Input: part model. Units: mm. Frame: model coordinates. Face numbers are marked on the shaded views. A direction names the side the tool comes from. Round coordinates to 2 decimals unless told otherwise and drop trailing zeros. Order: outer loops, then holes, each group sorted by start corner. A loop starts at its lowest first (then second) coordinate and runs counter-clockwise, first axis right, second up. Notation, with made-up numbers: M 74,-37.75 L 97,-37.75 A26 cw 97,-17.75 Z; hole C 57,60.25 d10. An arc over 180 degrees is marked long. One line per question, with ' | ' between items.
```python
from build123d import *

# Parameters (mm, degrees)
SKETCH_1_W         = 110
SKETCH_1_H         = 74
EXTRUDE_10_DEPTH   = 70
EXTRUDE_10_2_DEPTH = 70
EXTRUDE_10_3_DEPTH = 70
EXTRUDE_11_DEPTH   = 65
SKETCH_1_12_W      = 110
SKETCH_1_12_H      = 74
SKETCH_1_12_R      = 2
EXTRUDE_12_DEPTH   = 6


with BuildPart() as part:
    # Sketch 1 → Extrude 10 (new body)
    with BuildSketch(Plane.XY):
        Polygon((60.422680412, 44.278350515), (-55.577319588, 44.278350515), (-55.577319588, 38.278350515), (-55.577319588, -35.721649485), (-55.577319588, -41.721649485), (60.422680412, -41.721649485), (60.422680412, -35.721649485), (60.422680412, 38.278350515), align=None)
        with Locations((2.422680412, 1.278350515)):
            Rectangle(SKETCH_1_W, SKETCH_1_H, mode=Mode.SUBTRACT)
    extrude(amount=EXTRUDE_10_DEPTH)



with BuildPart() as body_2:
    # Sketch 1 → Extrude 10 2 (new body)
    with BuildSketch(Plane.XY):
        Polygon((66.422680412, 44.278350515), (63.422680412, 44.278350515), (63.422680412, 38.278350515), (63.422680412, -35.721649485), (63.422680412, -41.721649485), (66.422680412, -41.721649485), align=None)
    extrude(amount=EXTRUDE_10_2_DEPTH)


with BuildPart() as body_3:
    # Sketch 1 → Extrude 10 3 (new body)
    with BuildSketch(Plane.XY):
        Polygon((-58.577319588, 44.278350515), (-61.577319588, 44.278350515), (-61.577319588, -41.721649485), (-58.577319588, -41.721649485), (-58.577319588, -35.721649485), (-58.577319588, 38.278350515), align=None)
    extrude(amount=EXTRUDE_10_3_DEPTH)


with BuildPart() as part_1:
    add(part.part)

    add(body_2.part)  # Extrude 11 merges body 2

    add(body_3.part)  # Extrude 11 merges body 3
    # Sketch 1_11 → Extrude 11 (add)
    with BuildSketch(Plane.XY):
        Polygon((-58.577319588, 38.278350515), (-58.577319588, 44.278350515), (-55.577319588, 44.278350515), (-55.577319588, 38.278350515), (-55.577319588, -35.721649485), (-55.577319588, -41.721649485), (-58.577319588, -41.721649485), (-58.577319588, -35.721649485), align=None)
        Polygon((60.422680412, -35.721649485), (60.422680412, -41.721649485), (63.422680412, -41.721649485), (63.422680412, -35.721649485), (63.422680412, 38.278350515), (63.422680412, 44.278350515), (60.422680412, 44.278350515), (60.422680412, 38.278350515), align=None)
    extrude(amount=EXTRUDE_11_DEPTH)

    # Sketch 1_12 → Extrude 12 (add)
    with BuildSketch(Plane.XY):
        with Locations((2.422680412, 1.278350515)):
            Rectangle(SKETCH_1_12_W, SKETCH_1_12_H)
        with Locations((-45.701201979, -31.095897639)):
            Circle(SKETCH_1_12_R, mode=Mode.SUBTRACT)
        with Locations((50.546562804, -31.095897639)):
            Circle(SKETCH_1_12_R, mode=Mode.SUBTRACT)
        with Locations((50.546562804, 33.65259867)):
            Circle(SKETCH_1_12_R, mode=Mode.SUBTRACT)
        with Locations((-45.701201979, 33.65259867)):
            Circle(SKETCH_1_12_R, mode=Mode.SUBTRACT)
        with Locations((-45.701201979, -16.095897639)):
            Circle(SKETCH_1_12_R, mode=Mode.SUBTRACT)
        with Locations((-45.701201979, 18.65259867)):
            Circle(SKETCH_1_12_R, mode=Mode.SUBTRACT)
        with Locations((50.546562804, 18.65259867)):
            Circle(SKETCH_1_12_R, mode=Mode.SUBTRACT)
        with Locations((50.546562804, -16.095897639)):
            Circle(SKETCH_1_12_R, mode=Mode.SUBTRACT)
    extrude(amount=EXTRUDE_12_DEPTH)


solid = part_1.part
```
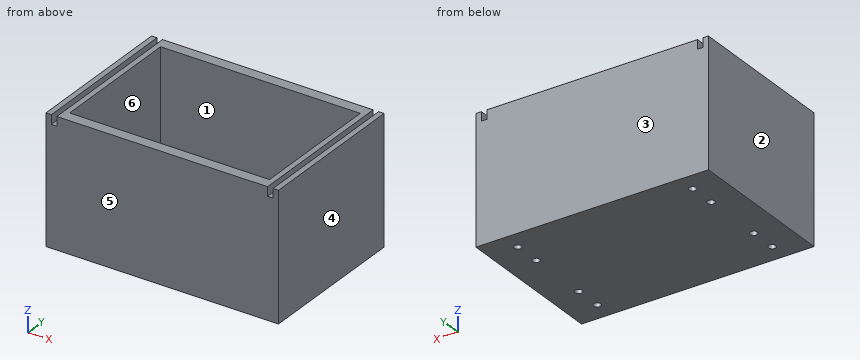
Item 1: Section query C-C, the plane x = 2. Return loops of the section in (y, z).
Report:
outline: M -41.72,0 L 44.28,0 L 44.28,70 L 38.28,70 L 38.28,6 L -35.72,6 L -35.72,70 L -41.72,70 Z
Item 2: First-contact query: pin 1 (2.5 mm diameter, centred on x = -57, y = 12, fed in from +Z); pin 2 (2.5 mm diameter, centred on x = -45.7, y = -16.1, fed in from -Z); pin 3 (6.5 mm diameter, centred on x = 50.55, y = -31.1, fed in from -Z); pin 4 (22 mm diameter, centred on x = 2.5, y = 10.5, fed in from +Z). Flat tips, straight axial feed; report the tip coordinate or a pass-through.
Report:
pin 1: z = 65 | pin 2: through | pin 3: z = 0 | pin 4: z = 6
Item 3: Access query for the marked faces 5 and 6. Directions: +Z, -Z, +X, -X, +Y, -Y. A direction counts if a zero-diameter tool reaches every point of the face in a straight line with its end or side. Return the directions, or none.
Report:
face 5: +Z, -Z, +X, -X, -Y | face 6: +Z
Item 4: Line query: line 1 along X through (y, z) = (27, 47.5); line 2 along Y through (x, z) = (4.5, 21); line 3 along Z through (x, y) = (38, 12.5). Output: solid intervals per line, ascending. Write a range as from..to.
Report:
line 1: -61.58..-52.58, 57.42..66.42 | line 2: -41.72..-35.72, 38.28..44.28 | line 3: 0..6
Item 5: Mould query, pull axis X, two halves, no side actions, for the marked faces 1, 2, 3 and 4. Classes: +X half, -X half, draft (parallel to the pull), parting line (faces both ways), or undercut.
Report:
face 1: undercut | face 2: -X half | face 3: draft | face 4: +X half
Item 6: Section query B-B, the plane y = 24. Return loops of the section in (x, z).
Report:
outline: M -61.58,0 L 66.42,0 L 66.42,70 L 63.42,70 L 63.42,65 L 60.42,65 L 60.42,70 L 57.42,70 L 57.42,6 L -52.58,6 L -52.58,70 L -55.58,70 L -55.58,65 L -58.58,65 L -58.58,70 L -61.58,70 Z
Item 7: Section query A-A, the plane z = 47. Return loops of the section in (x, y).
Report:
outline: M -61.58,-41.72 L 66.42,-41.72 L 66.42,44.28 L -61.58,44.28 Z; hole M -52.58,-35.72 L 57.42,-35.72 L 57.42,38.28 L -52.58,38.28 Z
